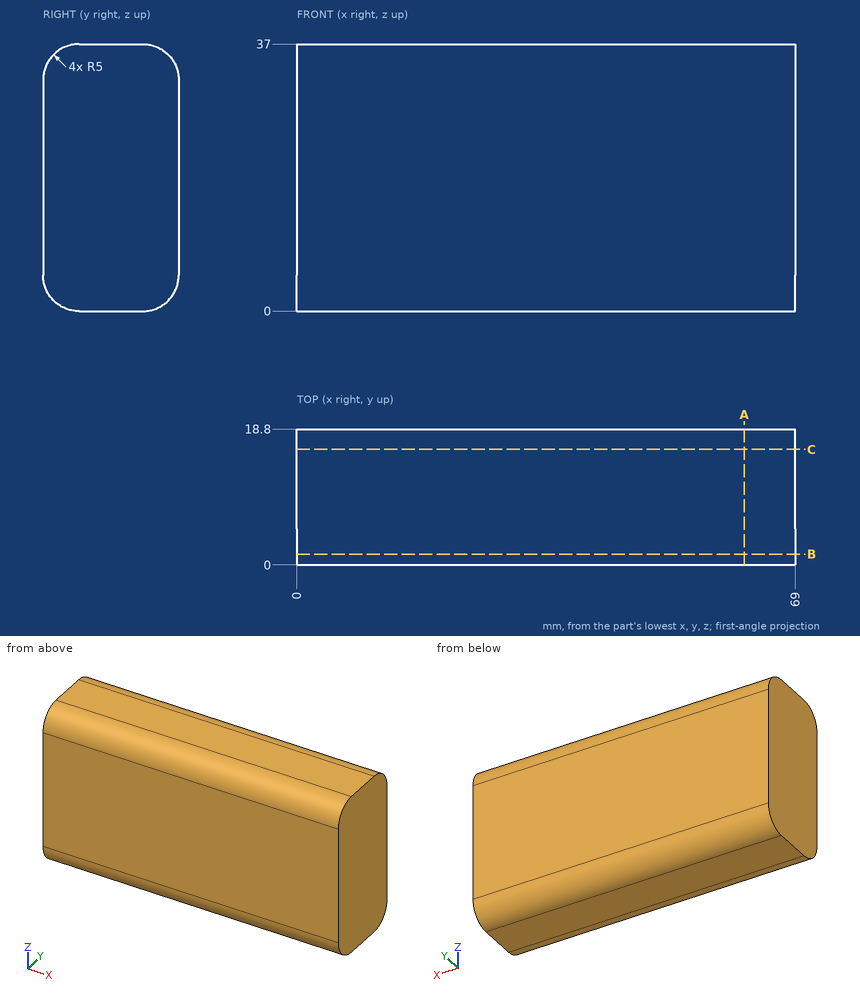
Study the drawing (mm; zero at the part's minimum x, y, z) and answer. Give positions to 0.01 mm unless a question says otherwise; leave off trailing zeros. Write each loop counter-clockwise with the first axis right and the second up, starting at its lowest first coordinate (ties: lowest second). Pieces come first, ordered by that corner, then holes. Notation, with made-up numbers: (26.25, -23) - (64.25, -23) arc R26 cw to (64.25, -7) - close; hole circle Ø6 at (32, -14). An arc over 180 degrees is marked (long way). Write item = value, one per line. Start each with the question number.
Item 1: Find section C-C (y = 16). Give the vertices of the cut face in (x, z).
Item 2: Find the intervals of material crossed by probe 1 along Z at (x, y) = (28, 4.75); probe 2 along Z at (x, y) = (23.5, 17.5); probe 3 along Y at (x, z) = (59.5, 34.5), in increasing order. Write a range as [from, to].
Item 3: Find section A-A (x = 62). Give the vertices of the cut face in (y, z), then the cut area to 3 significant figures.
Item 4: Find section B-B (y = 1.5). Give the vertices of the cut face in (x, z), then the cut area to 3 significant figures.
Response:
q1.outline = (0, 0.51) - (69, 0.51) - (69, 36.49) - (0, 36.49) - close
q2.probe_1 = [0.01, 36.99]
q2.probe_2 = [1.64, 35.36]
q2.probe_3 = [0.67, 18.13]
q3.outline = (0, 5) arc R5 ccw to (5, 0) - (13.8, 0) arc R5 ccw to (18.8, 5) - (18.8, 32) arc R5 ccw to (13.8, 37) - (5, 37) arc R5 ccw to (0, 32) - close
q3.area = 674 mm²
q4.outline = (0, 1.43) - (69, 1.43) - (69, 35.57) - (0, 35.57) - close
q4.area = 2,360 mm²
